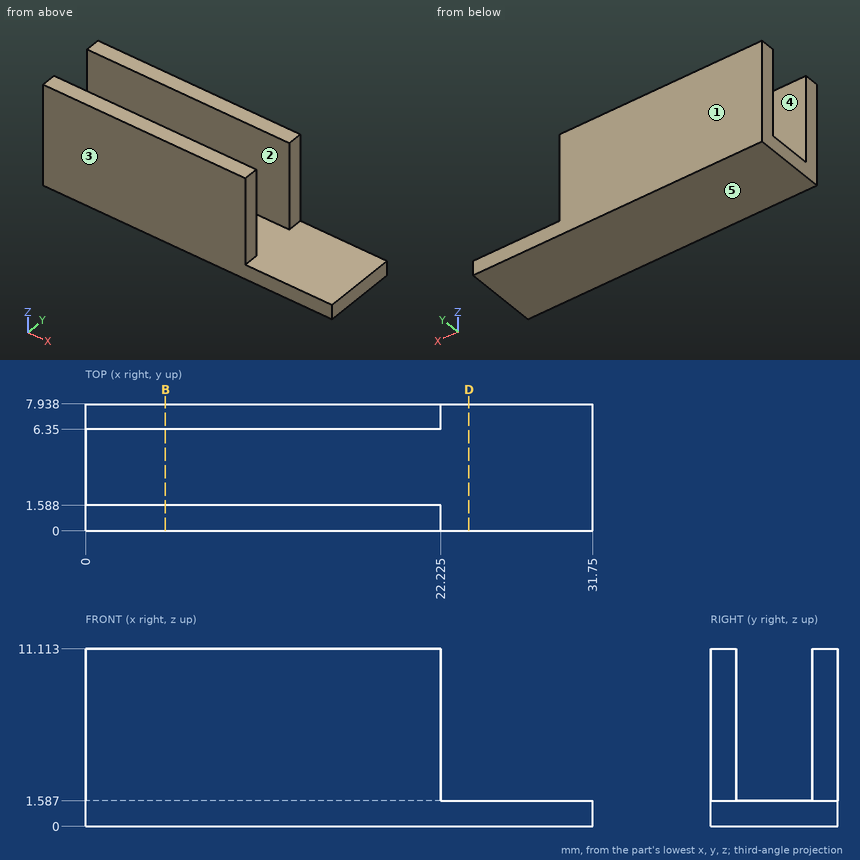
Study the drawing (mm; zero at the part's minimum x, y, z) and answer. A direction names the side the tool comes from. Give positions to 0.01 mm unless a question says otherwise; leave off trailing zeros. Loops run counter-clockwise (first coordinate to the right, second up) from the corner with the lowest first, then second, coordinate; pieces in that order, holes last. Notation, with made-up numbers: M -23,1 L 19,1 A24 cw 19,22 Z; hole C -39,55.25 d6. An arc over 180 degrees is marked long. Answer as CSV lines item,"result".
Item 1: Given pin 1 Ø1.3 at (y, z) = (7.5, 7) entering from +X (1 decimal); pin 2 Ø3 at (x, y) = (5.5, 4) entering from +Z; pin 3 Ø1 at (y, z) = (3.5, 8) entering from +X, each flat-ended and moving along its own axis, determine where each tip first touches the part or whether it passes through.
Values follow:
pin 1,"stops at x = 22.2"
pin 2,"stops at z = 1.59"
pin 3,"passes through"
Item 2: The part is cut by section D-D (x = 24). Give the vertices of the cut face in (y, z), and give its area (3 significant figures).
Values follow:
outline,"M 0,0 L 7.94,0 L 7.94,1.59 L 0,1.59 Z"
area,"12.6 mm^2"
Item 3: Which of the six approach directions +Z, -Z, +X, -X, +Y, -Y give full straight-line access (tool end or side, diameter ignored) to the marked faces 4 and 5?
Values follow:
face 4,"+Z, +X, -X"
face 5,"-Z, +X, -X, +Y, -Y"
Item 4: The mould has two halves that part along Y. Classify the marked faces 1, 2 and 3: released by +Y, released by -Y, zero draft, split by the parting line, or undercut.
Values follow:
face 1,"released by +Y"
face 2,"undercut"
face 3,"released by -Y"
Item 5: The part is cut by section B-B (x = 5). Give the vertices of the cut face in (y, z).
Values follow:
outline,"M 0,0 L 7.94,0 L 7.94,11.11 L 6.35,11.11 L 6.35,1.59 L 1.59,1.59 L 1.59,11.11 L 0,11.11 Z"
Item 6: Straight lines are drawn through the part: line 1 along Y through (x, z) = (20.5, 9); line 2 along Z through (x, y) = (22, 6); line 3 along X through (y, z) = (1, 10.25) (1 decimal). For each, find the intervals that lie inside material, in ascending order. Write a range as [from, to].
Values follow:
line 1,"y = [0, 1.59], [6.35, 7.94]"
line 2,"z = [0, 1.59]"
line 3,"x = [0, 22.2]"
